Geometry: final body of the model. Coordinates: model frame, mm. A direction names the side the tool comes from. Coordinates: 2 decimals unless noted, no trailing zeros. Write each loop counter-clockwise with the first axis right and the second up, starting at its lowest first coordinate (ties: lowest second). Pieces come first, ordered by that corner, then holes. Notation, with made-up numbers: (-6, -21.5) - (51, -21.5) arc R30 cw to (51, 11.5) - close; hole circle Ø4 at (22.25, -19.75). An arc over 180 degrees is marked (long way). Answer as a JSON object with one key per item and string values. Group by question number.
Item 1: Mould query, pull axis Y, two halves, no side actions, for faces 4 (the flat face through (39, 27.5, -112)), 5 (the flat face through (1, 25.5, -197)), 6 (the flat face through (17, 27, -200)). Classes: pulls with the +Y half, pulls with the -Y half, needs draft (parallel to the pull), parting line crosses it, or undercut.
Item 2: Section C-C on x = 49.5. Return loops of the section in (y, z).
Item 3: Set-up query: faces 1 (the flat face through (1, -25.5, -197)), 2 (the flat face through (17, 27, -80)), 3 (the flat face through (-1, 26.564, -193)). Return all of +Z, -Z, +X, -X, +Y, -Y with unobstructed straight access to the full face (end or side cutting, diameter ignored); none if empty.
Item 4: Section A-A on y = 19.5. Return loops of the section in (x, z).
Item 5: Section B-B on z = -140. Return loops of the section in (x, y), and give its area (3 significant figures).
Item 6: Section D-D on x = 0. State how many separate pieces and enclosed holes the cut face has, and give its area (3 significant figures).
Item 7: Line query: line 1 along Z through (x, y) = (0, -26); line 2 along Z through (x, y) = (0, 27.1); line 3 along Y through (x, z) = (42, -178). Output: solid intervals per line, ascending. Write a range as from..to.
```python
from build123d import *

# Parameters (mm, degrees)
SKETCH4_W               = 115
SKETCH4_H               = 55
SKETCH4_W_2             = 111
SKETCH4_H_2             = 51
FLAT_SURFACE_DEPTH      = 120
SKETCH9_R               = 45
CUT_EXTRUDE1_DEPTH      = 1
CUT_EXTRUDE1_DEPTH_BACK = 55
SKETCH10_W              = 4.252555104
SKETCH10_H              = 1.06386625
CUT_EXTRUDE2_DEPTH      = 111
MIRROR2_COPY_1_SKETCH_W = 4.252555104
MIRROR2_COPY_1_SKETCH_H = 1.06386625
MIRROR2_COPY_1_DEPTH    = 111


with BuildPart() as part:
    # Sketch4 → Flat-surface (new body)
    with BuildSketch(Plane(origin=(0, 0, -80), x_dir=(-1, 0, 0), z_dir=(0, 0, -1))):
        Rectangle(SKETCH4_W, SKETCH4_H)
        Rectangle(SKETCH4_W_2, SKETCH4_H_2, mode=Mode.SUBTRACT)
    extrude(amount=FLAT_SURFACE_DEPTH)

    # Sketch9 → Cut-Extrude1 (cut, two sides)
    with BuildSketch(Plane(origin=(0, 27.5, 0), x_dir=(1, 0, 0), z_dir=(0, 1, 0))) as cut_extrude1_sk:
        with Locations((0, 140)):
            Circle(SKETCH9_R)
    extrude(amount=CUT_EXTRUDE1_DEPTH, mode=Mode.SUBTRACT)
    extrude(cut_extrude1_sk.sketch, amount=-CUT_EXTRUDE1_DEPTH_BACK, mode=Mode.SUBTRACT)

    # Sketch10 → Cut-Extrude2 (cut)
    with BuildSketch(Plane(origin=(-55.5, 0, 0), x_dir=(0, 0, -1), z_dir=(1, 0, 0))):
        with Locations((87.126277552, 26.031933125)):
            Rectangle(SKETCH10_W, SKETCH10_H)
    cut_extrude2 = extrude(amount=CUT_EXTRUDE2_DEPTH, mode=Mode.SUBTRACT)

    # Mirror1: Cut-Extrude2 across plane
    add(cut_extrude2.mirror(Plane.ZX), mode=Mode.SUBTRACT)

    # Mirror2: Cut-Extrude2 across plane
    add(cut_extrude2.mirror(Plane(origin=(0, 0, -140), x_dir=(1, 0, 0), z_dir=(0, 0, -1))), mode=Mode.SUBTRACT)

    # Mirror2 copy 1 sketch → Mirror2 copy 1 (cut)
    with BuildSketch(Plane(origin=(-55.5, 0, -280), x_dir=(0, 0, 1), z_dir=(1, 0, 0))):
        with Locations((87.126277552, 26.031933125)):
            Rectangle(MIRROR2_COPY_1_SKETCH_W, MIRROR2_COPY_1_SKETCH_H)
    extrude(amount=MIRROR2_COPY_1_DEPTH, mode=Mode.SUBTRACT)


solid = part.part
```
Checks:
{
 "1": {"face 4": "pulls with the +Y half", "face 5": "undercut", "face 6": "needs draft"},
 "2": {"outline": "(-27.5, -200) - (-25.5, -200) - (-25.5, -195) - (-26.56, -195) - (-26.56, -190.75) - (-25.5, -190.75) - (-25.5, -89.25) - (-26.56, -89.25) - (-26.56, -85) - (-25.5, -85) - (-25.5, -80) - (-27.5, -80) - close; (25.5, -200) - (27.5, -200) - (27.5, -80) - (25.5, -80) - (25.5, -85) - (26.56, -85) - (26.56, -89.25) - (25.5, -89.25) - (25.5, -190.75) - (26.56, -190.75) - (26.56, -195) - (25.5, -195) - close"},
 "3": {"face 1": "+Z, -Z", "face 2": "+Z, +X, -X, +Y, -Y", "face 3": "none"},
 "4": {"outline": "(-57.5, -200) - (-55.5, -200) - (-55.5, -80) - (-57.5, -80) - close; (55.5, -200) - (57.5, -200) - (57.5, -80) - (55.5, -80) - close"},
 "5": {"outline": "(-57.5, -27.5) - (-45, -27.5) - (-45, -25.5) - (-55.5, -25.5) - (-55.5, 25.5) - (-45, 25.5) - (-45, 27.5) - (-57.5, 27.5) - close; (45, -27.5) - (57.5, -27.5) - (57.5, 27.5) - (45, 27.5) - (45, 25.5) - (55.5, 25.5) - (55.5, -25.5) - (45, -25.5) - close", "area": "304 mm^2"},
 "6": {"separate pieces": "4", "enclosed holes": "0", "area": "102 mm^2"},
 "7": {"line 1": "-200..-195, -190.75..-185, -95..-89.25, -85..-80", "line 2": "-200..-185, -95..-80", "line 3": "-27.5..-25.5, 25.5..27.5"}
}
